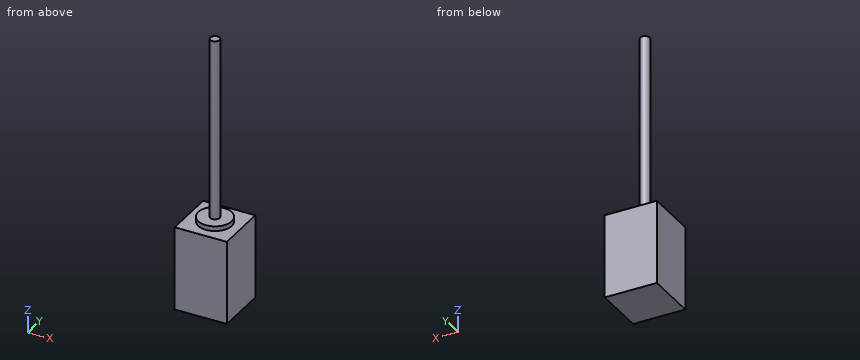
```python
from build123d import *

# Parameters (mm, degrees)
F0_W     = 28
F0_H     = 28
F0_R     = 9
F0_R_2   = 2.5
F1_DEPTH = 45
F2_DEPTH = 100
F3_DEPTH = 2.54


with BuildPart() as f1:
    # F0 (on Top) → F1 (new body)
    with BuildSketch(Plane.XY):
        Rectangle(F0_W, F0_H)
        Circle(F0_R, mode=Mode.SUBTRACT)
        Circle(F0_R)
        Circle(F0_R_2, mode=Mode.SUBTRACT)
        Circle(F0_R_2)
    extrude(amount=-F1_DEPTH)

    # F0 (on Top) → F2 (join)
    with BuildSketch(Plane.XY):
        Circle(F0_R_2)
    extrude(amount=F2_DEPTH)

    # F0 (on Top) → F3 (join)
    with BuildSketch(Plane.XY):
        Circle(F0_R)
        Circle(F0_R_2, mode=Mode.SUBTRACT)
    extrude(amount=F3_DEPTH)


solid = f1.part
```
Read the model definition and answer for the solid it produces. Units are mm, in the model's axes. Coordinates: 2 decimals unless noted, no trailing zeros. Write each loop counter-clockwise with the first axis right and the second up, starting at its lowest first coordinate (ties: lowest second). Pieces come first, ordered by that corner, then holes. Notation, with made-up numbers: (-35.75, 54) -> (5.25, 54) arc R22 ccw to (5.25, 61) -> close; hole circle Ø11 at (-24.75, 20.5). An arc over 180 degrees is marked (long way). Return JSON: item names as keys, results as strings.
1. A cutting plane is placed at D-D (y = -10.25). Determine the outline of the cut face in (x, z).
Found:
{"outline": "(-14, -45) -> (14, -45) -> (14, 0) -> (-14, 0) -> close"}
2. Find the intervals of material crossed by line 1 along Z through (x, y) = (5, 6); line 2 along Z through (x, y) = (-11.5, 11); line 3 along Y through (x, z) = (-2.25, 46), in increasing order. Write a range as from..to.
Found:
{"line 1": "-45..2.54", "line 2": "-45..0", "line 3": "-1.09..1.09"}
3. A cutting plane is placed at A-A (x = 0). Determine the outline of the cut face in (y, z), and give its area (3 significant figures).
Found:
{"outline": "(-14, -45) -> (14, -45) -> (14, 0) -> (9, 0) -> (9, 2.54) -> (2.5, 2.54) -> (2.5, 100) -> (-2.5, 100) -> (-2.5, 2.54) -> (-9, 2.54) -> (-9, 0) -> (-14, 0) -> close", "area": "1,790 mm2"}
4. Each of these flat-tipped pins is pushed along its axis until it touches: P1, Ø2, axis at x = -11, y = 9, coming from the +Z side; P2, Ø10, axis at x = 3.5, y = 0, coming from the +Z side. Where does it stop, or does it pass through?
Found:
{"P1": "z = 0", "P2": "z = 100"}
5. A cutting plane is placed at C-C (z = 10). Determine the outline of the cut face in (x, y), and give its area (3 significant figures).
Found:
{"outline": "circle Ø5 at (0, 0)", "area": "19.6 mm2"}
